Part print with two shaded views. Sizes in mm from the minimum x, y, z corner. A direction names the side the tool comes from. Round coordinates to 2 decimals unless told otherwise and drop trailing zeros. Write each loop counter-clockwise with the first axis right and the second up, starting at its lowest first coordinate (ties: lowest second). Pieces come first, ordered by that corner, then holes. Notation, with made-up numbers: M -31,36.5 L 4,36.5 A18 ccw 4,42.5 Z; hole C 71,-38 d7. An arc over 180 degrees is marked long. One line per question, with ' | ' between items. Start each with the question number.
1) Wall check: probe 1 along Z at (x, y) = (3, 7); probe 2 along Y at (x, z) = (5.5, 10.75); probe 3 along Y at (x, z) = (13.75, 2). Give the ranges that are in metal, low to high. Write a range as [from, to].
2) Tool access for the marked faces 1 and 2: list every direction of +Z, -Z, +X, -X, +Y, -Y with a clear straight run to the whole face (end or side of a thin tool).
3) Drop flat-ended pins along their axis: pin 1 Ø2 at (x, z) = (3.5, 9) entering from -Y; pin 2 Ø6 at (y, z) = (4, 4) entering from -X; pin 3 Ø4 at (x, y) = (4, 12.5) entering from +Z; pin 4 Ø1 at (y, z) = (9, 7) entering from +X. Give the stop position or say it passes through.
4) Saw through at C-C (z = 15.25). List the corners of the cut face in (x, y) (3 decimals), plus the area to 3 significant figures.
5) Saw through at A-A (x = 7.5). List the corners of the cut face in (y, z) (3 decimals).
6) Saw through at D-D (z = 3.5). List the corners of the cut face in (x, y), plus the area to 3 significant figures.
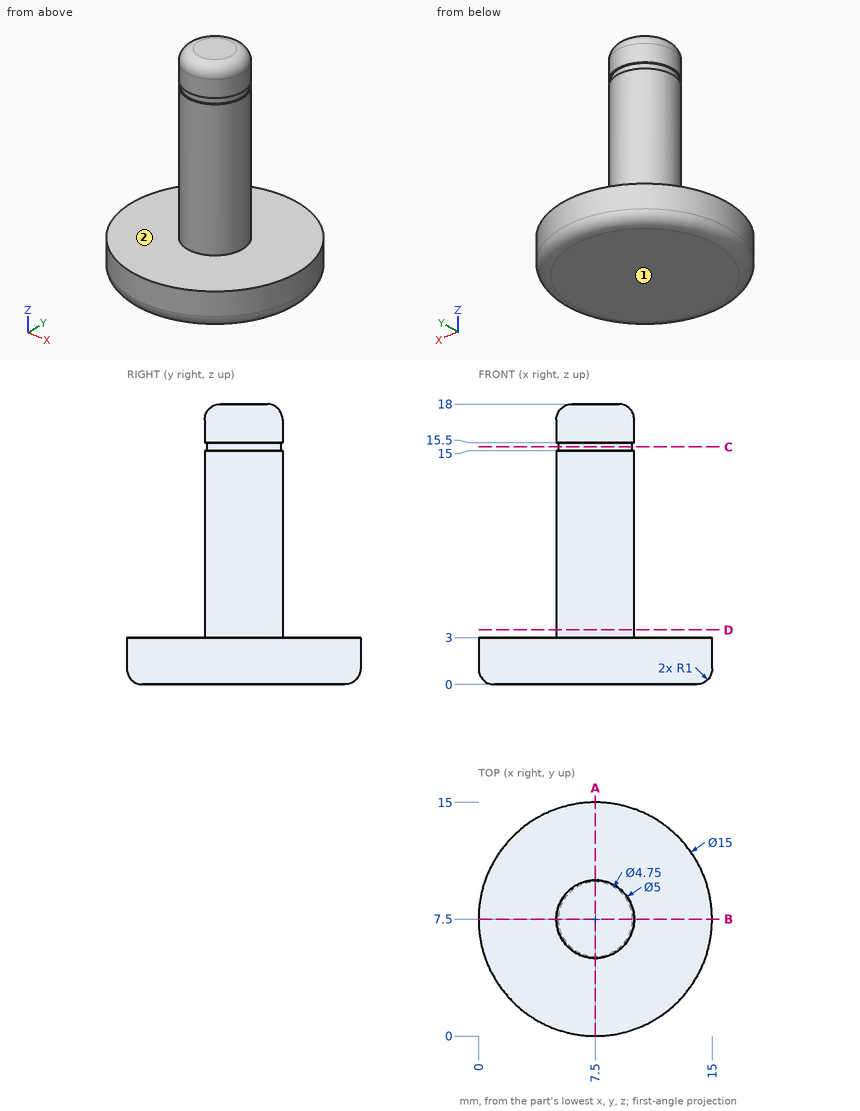
Answer key:
1) probe 1: z = [0, 3] | probe 2: y = [6, 9] | probe 3: y = [3.35, 11.65]
2) face 1: -Z, +X, -X, +Y, -Y | face 2: +Z
3) pin 1: passes through | pin 2: stops at x = 0.03 | pin 3: stops at z = 3 | pin 4: stops at x = 9.79
4) outline: C 7.5,7.5 d4.75 | area: 17.7 mm2
5) outline: M 0,1 A1 ccw 1,0 L 14,0 A1 ccw 15,1 L 15,3 L 10,3 L 10,15 L 9.875,15 L 9.875,15.5 L 10,15.5 L 10,17 A1 ccw 9,18 L 6,18 A1 ccw 5,17 L 5,15.5 L 5.125,15.5 L 5.125,15 L 5,15 L 5,3 L 0,3 Z
6) outline: C 7.5,7.5 d5 | area: 19.6 mm2
